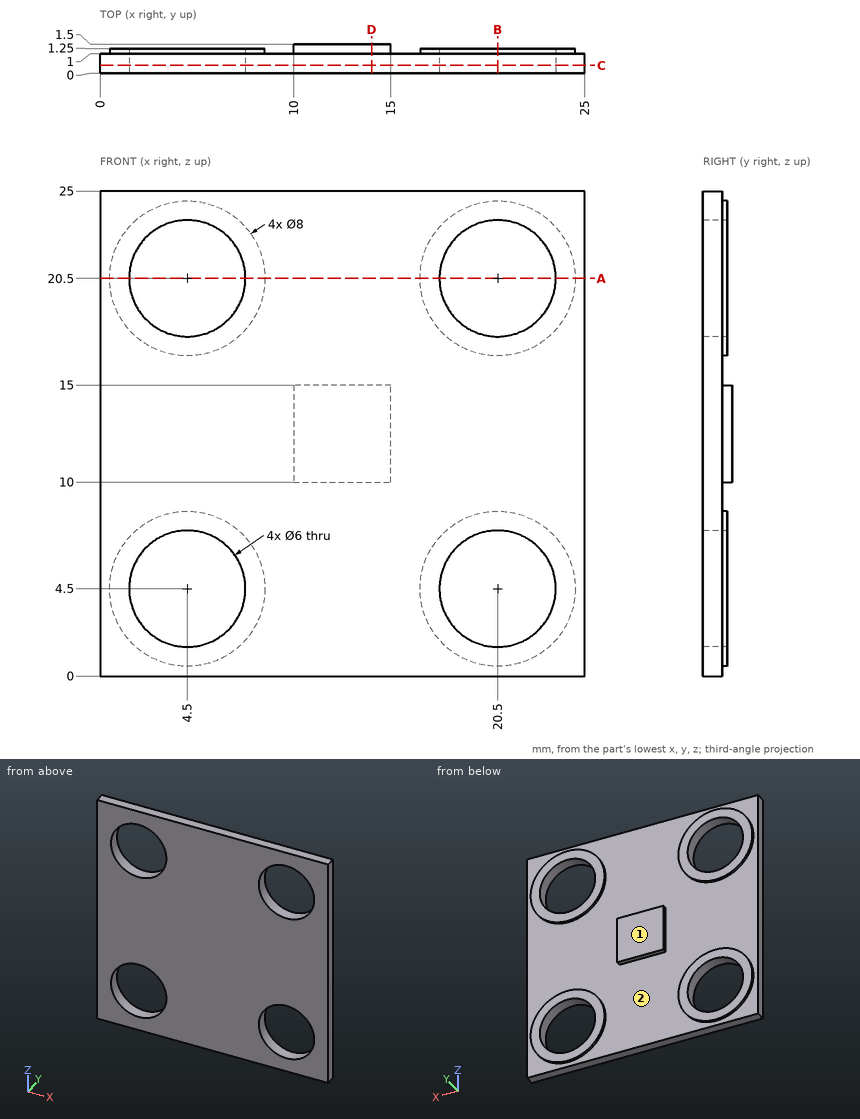
Source: three-view drawing plus pictorial views. Frame: mm from the lowest corner of the part. Coordinates: 2 decimals unless noted, no trailing zeros. Loops run counter-clockwise (first coordinate to the right, second up) from the corner with the lowest first, then second, coordinate; pieces in that order, holes last. Notation, with made-up numbers: (58, 73) -> (96, 73) arc R6 cw to (96, 81) -> close; hole circle Ø7 at (63.5, 13). An arc over 180 degrees is marked (long way). Write each question's results on one line, items separated by ' | '. Start each with the question number.
Q1. Pull-direction query (X, two-part tool) for the marked faces 1 and 2; classes: released by +X, released by -X, zero draft, split by the parting line, or undercut.
Q2. Section D-D, the plane x = 14. Return the cut outline in (y, z).
Q3. Section C-C, the plane y = 0.4. Return the cut outline in (x, z), plus the area to 3 significant figures.
Q4. Pin query (flat end, axial travel): pin 1 (9.5 mm diameter, centred on x = 4.5, z = 20.5, fed in from +Y); pin 2 (1 mm diameter, centred on x = 9, z = 22, fed in from +Y). Return the tip coordinate at first contact, or that it passes through.
Q5. Ray query, line 1 (X direction, y = 0.3, z = 20.5); line 2 (Z direction, x = 22.5, y = 0.45). Return the intervals inside material, ascending. Write a range as from..to.
Q6. Section B-B, the plane x = 20.5. Return the cut outline in (y, z), plus the area to 3 significant figures.
Q7. Section A-A, the plane z = 20.5. Return the cut outline in (x, y), plus the area to 3 significant figures.
Found:
1) face 1: zero draft | face 2: undercut
2) outline: (0, 0) -> (1, 0) -> (1, 10) -> (1.5, 10) -> (1.5, 15) -> (1, 15) -> (1, 25) -> (0, 25) -> close
3) outline: (0, 0) -> (25, 0) -> (25, 25) -> (0, 25) -> close; hole circle Ø6 at (4.5, 4.5); hole circle Ø6 at (4.5, 20.5); hole circle Ø6 at (20.5, 4.5); hole circle Ø6 at (20.5, 20.5) | area: 512 mm2
4) pin 1: y = 1.25 | pin 2: y = 1
5) line 1: 0..1.5, 7.5..17.5, 23.5..25 | line 2: 0..2.26, 6.74..18.26, 22.74..25
6) outline: (0, 0) -> (1, 0) -> (1, 0.5) -> (1.25, 0.5) -> (1.25, 1.5) -> (0, 1.5) -> close; (0, 7.5) -> (1.25, 7.5) -> (1.25, 8.5) -> (1, 8.5) -> (1, 16.5) -> (1.25, 16.5) -> (1.25, 17.5) -> (0, 17.5) -> close; (0, 23.5) -> (1.25, 23.5) -> (1.25, 24.5) -> (1, 24.5) -> (1, 25) -> (0, 25) -> close | area: 14.0 mm2
7) outline: (0, 0) -> (1.5, 0) -> (1.5, 1.25) -> (0.5, 1.25) -> (0.5, 1) -> (0, 1) -> close; (7.5, 0) -> (17.5, 0) -> (17.5, 1.25) -> (16.5, 1.25) -> (16.5, 1) -> (8.5, 1) -> (8.5, 1.25) -> (7.5, 1.25) -> close; (23.5, 0) -> (25, 0) -> (25, 1) -> (24.5, 1) -> (24.5, 1.25) -> (23.5, 1.25) -> close | area: 14.0 mm2
